CAD build for the part. Positions are in the model's coordinates, mm. Give positions to 0.01 mm unless a question says otherwise; leave off trailing zeros. Order: outer loops, then holes, each group sorted by start corner. A loop starts at its lowest first (then second) coordinate and runs counter-clockwise, first axis right, second up. Notation, with made-up numbers: (59, 5) -> (68, 5) arc R12 ccw to (68, 13) -> close; hole circle Ø6 at (81, 8.25). An arc over 180 degrees is marked (long way). Answer as CSV lines item,"result".
```python
from build123d import *

# Parameters (mm, degrees)
SKETCH1_R           = 2.5
BOSS_EXTRUDE1_DEPTH = 4


with BuildPart() as part:
    # Sketch1 → Boss-Extrude1 (new body)
    with BuildSketch(Plane(origin=(0, 0, 0), x_dir=(1, 0, 0), z_dir=(0, 1, 0))):
        Polygon((-185, -69), (-185, 69), (-164, 69), (-164, 90), (185, 90), (185, -69), (-164, -69), align=None)
        with Locations((-155, 80)):
            Circle(SKETCH1_R, mode=Mode.SUBTRACT)
        with Locations((0, 80)):
            Circle(SKETCH1_R, mode=Mode.SUBTRACT)
        with Locations((155, 80)):
            Circle(SKETCH1_R, mode=Mode.SUBTRACT)
    extrude(amount=BOSS_EXTRUDE1_DEPTH)


solid = part.part
```
1) Band-saw the part on A-A, the plane z = -72.5. Write the cut outline in (x, y).
Data:
outline,"(-164, 0) -> (185, 0) -> (185, 4) -> (-164, 4) -> close"
2) Wall check: line 1 along X through (y, z) = (2.7, -80); line 2 along X through (y, z) = (0.25, -80.5); line 3 along Z through (x, y) = (0, 2.1). Give the ranges that are in metal, low to high. Write a range as [from, to].
Data:
line 1,"x = [-164, -157.5], [-152.5, -2.5], [2.5, 152.5], [157.5, 185]"
line 2,"x = [-164, -157.45], [-152.55, -2.45], [2.45, 152.55], [157.45, 185]"
line 3,"z = [-90, -82.5], [-77.5, 69]"
3) Pin check, flat tips, straight feed: P1, Ø1.2, axis at x = -176.5, y = 2, coming from the -Z side; P2, Ø3, axis at x = -155, z = -80, coming from the -Y side. Stop position of each tip, or through.
Data:
P1,"stops at z = -69"
P2,"passes through"
